Geometry: final body of the model. Coordinates: model frame, mm. A direction names the side the tool comes from. Round coordinates to 2 decimals unless told otherwise and drop trailing zeros. Order: outer loops, then holes, each group sorted by start corner. A loop starts at its lowest first (then second) coordinate and runs counter-clockwise, first axis right, second up. Notation, with made-up numbers: (62, -13.75) - (106, -13.75) arc R22 cw to (106, 23.25) - close; hole circle Ø6 at (-17.5, -18). An arc over 180 degrees is marked (long way). Put each result on its own line as item: value. Start each with the question number.
(1) Section C-C (x = 105.5). Output: boundary loops of the cut face in (y, z), and give its area (3 significant figures).
(2) Section A-A (y = 0). Output: boundary loops of the cut face in (x, z), and give its area (3 significant figures).
(3) Section B-B (z = 5.75). Output: boundary loops of the cut face in (x, y), and give its area (3 significant figures).
(4) Pin query (flat end, axial travel): P1, Ø1, axis at x = 205.5, z = 3, coming from the +Y side; P2, Ø7.5, axis at x = 25, y = 25, coming from the +Z side. Return the tip coordinate at first contact, or that it passes through.
(5) Section D-D (y = 25). Output: boundary loops of the cut face in (x, z), and give its area (3 significant figures).
(6) Material intervals for L1, parallel to X at y = -25, z = 8; L2, parallel to X at y = 0.5, z = 0.5; L3, parallel to Y at x = 106, z = 8.25, sorted ascending. Write a range as [from, to].
(7) Pull-direction query (Y, two-part tool) for faces 1 (the face through (29.214, -24.447, 5.07)), 2 (the face through (123, -9, 10)), 3 (the face through (123, 45, 5)); classes: released by +Y, released by -Y, zero draft, split by the parting line, or undercut.
(8) Access query for faces 4 (the face through (160.31, -0.11, 5.07)), 5 (the face through (123, -45, 5)). Directions: +Z, -Z, +X, -X, +Y, -Y. A direction counts if a zero-diameter tool reaches every point of the face in a straight line with its end or side. Return the directions, or none.
from build123d import *

# Parameters (mm, degrees)
PAD002_DEPTH    = 250
SKETCH004_R     = 4.25
HOLE_DEPTH      = 25
POCKET002_DEPTH = 10.001


with BuildPart() as part:
    # Sketch003 → Pad002 (new body)
    with BuildSketch(Plane.YZ):
        Polygon((-40, 10), (40, 10), (50, 0), (-50, 0), align=None)
    extrude(amount=PAD002_DEPTH)

    # Sketch004 (on Face2 of Pad002) → Hole (cut)
    with BuildSketch(Plane(origin=(0, 0, 10), x_dir=(0, -1, 0), z_dir=(0, 0, 1))):
        with Locations((-25, 25)):
            Circle(SKETCH004_R)
        with Locations((25, 25)):
            Circle(SKETCH004_R)
        with Locations((25, 225)):
            Circle(SKETCH004_R)
        with Locations((-25, 225)):
            Circle(SKETCH004_R)
    extrude(amount=-HOLE_DEPTH, mode=Mode.SUBTRACT)

    # Sketch005 (on Face3 of Hole) → Pocket002 (cut, through all)
    with BuildSketch(Plane(origin=(0, 0, 10), x_dir=(0, -1, 0), z_dir=(0, 0, 1))):
        with BuildLine():
            ThreePointArc((5, 155.310546), (0, 160.310546), (-5, 155.310546))
            Line((-5, 155.310546), (-5, 94.689454))
            ThreePointArc((-5, 94.689454), (0, 89.689454), (5, 94.689454))
            Line((5, 155.310546), (5, 94.689454))
        make_face()
    extrude(amount=-POCKET002_DEPTH, mode=Mode.SUBTRACT)


solid = part.part
Checks:
1. outline: (-50, 0) - (-5, 0) - (-5, 10) - (-40, 10) - close; (5, 0) - (50, 0) - (40, 10) - (5, 10) - close
1. area: 800 mm²
2. outline: (0, 0) - (89.69, 0) - (89.69, 10) - (0, 10) - close; (160.31, 0) - (250, 0) - (250, 10) - (160.31, 10) - close
2. area: 1,790 mm²
3. outline: (0, -44.25) - (250, -44.25) - (250, 44.25) - (0, 44.25) - close; hole circle Ø8.5 at (25, -25); hole circle Ø8.5 at (25, 25); hole (94.69, -5) - (155.31, -5) arc R5 ccw to (155.31, 5) - (94.69, 5) arc R5 ccw to start; hole circle Ø8.5 at (225, -25); hole circle Ø8.5 at (225, 25)
3. area: 21,200 mm²
4. P1: stops at y = 47.5
4. P2: passes through
5. outline: (0, 0) - (20.75, 0) - (20.75, 10) - (0, 10) - close; (29.25, 0) - (220.75, 0) - (220.75, 10) - (29.25, 10) - close; (229.25, 0) - (250, 0) - (250, 10) - (229.25, 10) - close
5. area: 2,330 mm²
6. L1: x = [0, 20.75], [29.25, 220.75], [229.25, 250]
6. L2: x = [0, 89.71], [160.29, 250]
6. L3: y = [-41.75, -5], [5, 41.75]
7. face 1: undercut
7. face 2: zero draft
7. face 3: released by +Y
8. face 4: +Z, -Z
8. face 5: +Z, +X, -X, -Y
